```python
from build123d import *

# Parameters (mm, degrees)
BOSS_EXTRUDE1_DEPTH = 170
FILLET2_R           = 3
SKETCH2_R           = 2.1
CUT_EXTRUDE1_DEPTH  = 8
CUT_EXTRUDE2_START  = -12
CUT_EXTRUDE2_DEPTH  = 9
FILLET3_R           = 2
FILLET4_R           = 2


with BuildPart() as part:
    # Sketch1 → Boss-Extrude1 (new body)
    with BuildSketch(Plane.XY):
        Polygon((13, -6), (13, 0), (0, 0), (0, -8), (6, -8), (10, -12), (21, -12), (21, -6), align=None)
    extrude(amount=-BOSS_EXTRUDE1_DEPTH)

    # Fillet2
    fillet2_edges = [part.edges().sort_by_distance(p)[0] for p in [
        (13, -6, -85),
    ]]
    fillet(fillet2_edges, radius=FILLET2_R)

    # Sketch2 → Cut-Extrude1 (cut)
    with BuildSketch(Plane(origin=(0, 0, 0), x_dir=(1, 0, 0), z_dir=(0, 1, 0))):
        with Locations(Location((5, 10, 0), (0, 0, 270))):
            Circle(SKETCH2_R)
        with Locations(Location((5, 160, 0), (0, 0, 270))):
            Circle(SKETCH2_R)
    extrude(amount=-CUT_EXTRUDE1_DEPTH, mode=Mode.SUBTRACT)

    # Sketch3 → Cut-Extrude2 (cut)
    with BuildSketch(Plane(origin=(0, 0, 0), x_dir=(1, 0, 0), z_dir=(0, 1, 0)).offset(CUT_EXTRUDE2_START)):
        Polygon((1.55, 11.991858429), (1.55, 8.008141571), (5, 6.016283143), (8.45, 8.008141571), (8.45, 11.991858429), (5, 13.983716857), align=None)
        Polygon((1.55, 161.991858429), (1.55, 158.008141571), (5, 156.016283143), (8.45, 158.008141571), (8.45, 161.991858429), (5, 163.983716857), align=None)
    extrude(amount=CUT_EXTRUDE2_DEPTH, mode=Mode.SUBTRACT)

    # Fillet3
    fillet3_edges = [part.edges().sort_by_distance(p)[0] for p in [
        (21, -6, -85),
        (21, -12, -85),
    ]]
    fillet(fillet3_edges, radius=FILLET3_R)

    # Fillet4
    fillet4_edges = [part.edges().sort_by_distance(p)[0] for p in [
        (10, -12, -85),
        (6, -8, -166.703183294),
        (6, -8, -85),
        (6, -8, -3.296816706),
    ]]
    fillet(fillet4_edges, radius=FILLET4_R)


solid = part.part
```
Source: CAD feature listing. Evaluate the final solid. Frame: model axes, mm. A direction names the side the tool comes from. Coordinates: 2 decimals unless noted, no trailing zeros. Loops run counter-clockwise (first coordinate to the right, second up) from the corner with the lowest first, then second, coordinate; pieces in that order, holes last. Notation, with made-up numbers: (66.5, -31) -> (82.5, -31) arc R30 ccw to (82.5, 2) -> close; hole circle Ø10 at (10.25, 55.5). An arc over 180 degrees is marked (long way). One line per item, written item: value. Start each with the question number.
Q1. Line query: line 1 along X through (y, z) = (-0.8, -10); line 2 along Y through (x, z) = (2.5, -79.5); line 3 along Y through (x, z) = (10.75, -129). Output: solid intervals per line, ascending.
Q2. Mould query, pull axis X, two halves, no side actions, for faces 1 (the face through (10, -6, -170)), 2 (the face through (8, -10, -84)), 3 (the face through (6.5, -3, -158.3)), 4 (the face through (5.631, -1.479, -157.997)). Classes: pulls with the +X half, pulls with the -X half, needs draft (parallel to the pull), parting line crosses it, or undercut.
Q3. Section query A-A, the plane z = -10. Return the cut outline in (x, y).
Q4. Contact query for flat-ended pins moving along their axis: P1, Ø7.5, axis at x = 5.5, z = -11.5, coming from the -Y side; P2, Ø3.5, axis at x = 17, z = -52.5, coming from the +Y side; P3, Ø7.5, axis at x = 5, z = -158, coming from the -Y side. Output: stop coordinate, or through.
Q5. Set-up query: faces 5 (the face through (1.55, -6, -10)), 6 (the face through (13.86, -5.1, -86.19)), 7 (the face through (3, -8, -84)). Return all of +Z, -Z, +X, -X, +Y, -Y with unobstructed straight access to the full face (end or side cutting, diameter ignored); none if empty.
Q6. Section query B-B, the plane z = -83.5. Return the cut outline in (x, y).
Results:
1. line 1: 0 to 2.9, 7.1 to 13
1. line 2: -8 to 0
1. line 3: -12 to 0
2. face 1: needs draft
2. face 2: pulls with the -X half
2. face 3: undercut
2. face 4: undercut
3. outline: (0, -8) -> (1.55, -8) -> (1.55, -3) -> (2.9, -3) -> (2.9, 0) -> (0, 0) -> close; (7.1, -3) -> (8.45, -3) -> (8.45, -10.45) -> (9.41, -11.41) arc R2 ccw to (10.83, -12) -> (19, -12) arc R2 ccw to (21, -10) -> (21, -8) arc R2 ccw to (19, -6) -> (16, -6) arc R3 cw to (13, -3) -> (13, 0) -> (7.1, 0) -> close
4. P1: y = -11.25
4. P2: y = -5.9
4. P3: y = -10.75
5. face 5: -Y
5. face 6: +Z, -Z, +X, +Y
5. face 7: +Z, -Z, -X, -Y
6. outline: (0, -8) -> (5.17, -8) arc R2 cw to (6.59, -8.59) -> (9.41, -11.41) arc R2 ccw to (10.83, -12) -> (19, -12) arc R2 ccw to (21, -10) -> (21, -8) arc R2 ccw to (19, -6) -> (16, -6) arc R3 cw to (13, -3) -> (13, 0) -> (0, 0) -> close
